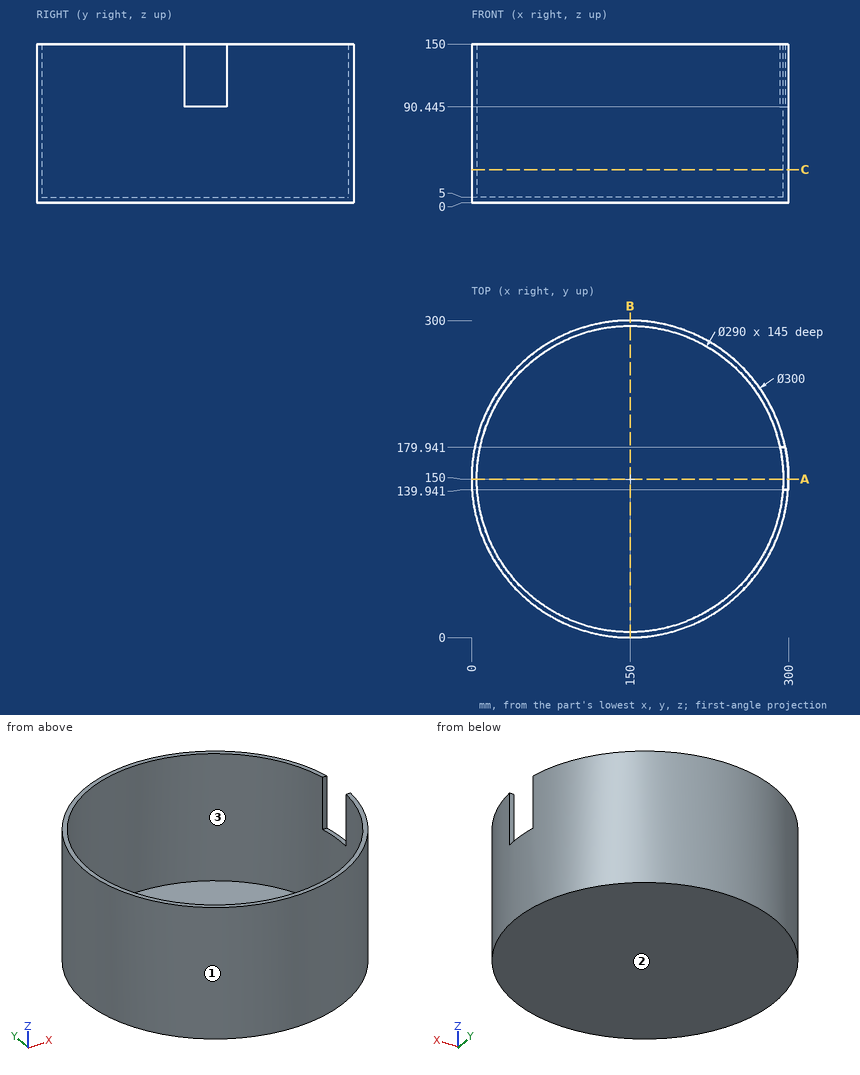
Input: dimensioned drawing with shaded views. Units: mm. Origin: part minimum x, y, z. Coordinates: 2 decimals unless noted, no trailing zeros. Loops run counter-clockwise (first coordinate to the right, second up) from the corner with the lowest first, then second, coordinate; pieces in that order, holes last. Notation, with made-up numbers: (-28, 4.5) -> (19, 4.5) arc R6 cw to (19, 9.5) -> close; hole circle Ø7 at (42.25, 62). An arc over 180 degrees is marked (long way). Use a Markdown table: item, result. Add a question column.
(1) Section query A-A, the plane y = 150. Return loops of the section in (x, z) (1 decimal), plus the area to 3 significant figures.
(2) Pin query (flat end, axial travel): pin 1 Ø2 at (x, y) = (165, 152) entering from +Z; pin 2 Ø10 at (y, z) = (124, 25.5) entering from +X; pin 3 Ø3 at (y, z) = (205, 51.5) entering from -X (1 decimal); pin 4 Ø1.5 at (x, y) = (51, 254) entering from -Z. Return the tip coordinate at first contact, or that it passes through.
(3) Section query B-B, the plane x = 150. Return loops of the section in (y, z), plus the area to 3 significant figures.
(4) Section query C-C, the plane z = 31. Return loops of the section in (x, y).
(5) Mould query, pull axis Y, two halves, no side actions, for the marked faces 1, 2 and 3. Classes: pulls with the +Y half, pulls with the -Y half, needs draft (parallel to the pull), parting line crosses it, or undercut.
(6) Line query: line 1 along Y through (x, z) = (150, 47); line 2 along Z through (x, y) = (161.5, 174). Output: solid intervals per line, ascending.
Answer:
| question | item | result |
|---|---|---|
| 1 | outline | (0, 0) -> (300, 0) -> (300, 90.4) -> (295, 90.4) -> (295, 5) -> (5, 5) -> (5, 150) -> (0, 150) -> close |
| 1 | area | 2,650 mm^2 |
| 2 | pin 1 | stops at z = 5 |
| 2 | pin 2 | stops at x = 298.52 |
| 2 | pin 3 | stops at x = 9.9 |
| 2 | pin 4 | stops at z = 0 |
| 3 | outline | (0, 0) -> (300, 0) -> (300, 150) -> (295, 150) -> (295, 5) -> (5, 5) -> (5, 150) -> (0, 150) -> close |
| 3 | area | 2,950 mm^2 |
| 4 | outline | circle Ø300 at (150, 150); hole circle Ø290 at (150, 150) |
| 5 | face 1 | parting line crosses it |
| 5 | face 2 | needs draft |
| 5 | face 3 | undercut |
| 6 | line 1 | y = 0 to 5, 295 to 300 |
| 6 | line 2 | z = 0 to 5 |
